Autodesk Inventor part; units mm, degrees
ref_plane "YZ Plane" through (0, 0, 0) normal (1, 0, 0) x (0, 1, 0)
ref_plane "XZ Plane" through (0, 0, 0) normal (0, 1, 0) x (-1, 0, 0)
ref_plane "XY Plane" through (0, 0, 0) normal (0, 0, 1) x (1, 0, 0)
sketch "Szkic1" plane through (0, 0, 0) normal (0, 1, 0) x (-1, 0, 0)
  line L0 (-100, 0) -> (-100, -48)
  line L1 (-11, -7.5) -> (0, -7.5)
  line L2 (-11, -40.5) -> (0, -40.5)
  line L3 (-16, 0) -> (-16, -10.5)
  line L4 (-16, -10.5) -> (-11, -10.5)
  line L5 (-16, -48) -> (-16, -37.5)
  line L6 (-16, -37.5) -> (-11, -37.5)
  line L7 (-11, -21.5) -> (-16, -21.5)
  line L8 (-16, -21.5) -> (-16, -26.5)
  line L9 (-16, -26.5) -> (-11, -26.5)
  line L10 (0, -7.5) -> (0, -14.4549)
  line L11 (0, -40.5) -> (0, -37.5)
  line L12 (0, -7.5) -> (0, -10.5)
  line L13 (0, -10.5) -> (-11, -21.5)
  line L14 (-11, -26.5) -> (0, -37.5)
  line L15 (-100, 0) -> (-100, -48)
  line L16 (-100, 0) -> (-16, 0)
  line L17 (-16, -10.5) -> (-16, 0)
  line L18 (-16, -10.5) -> (-11, -10.5)
  line L19 (-11, -10.5) -> (-11, -7.5)
  line L20 (-11, -7.5) -> (0, -7.5)
  line L21 (0, -7.5) -> (0, -10.5)
  line L22 (0, -10.5) -> (-11, -21.5)
  line L23 (-11, -21.5) -> (-16, -21.5)
  line L24 (-16, -21.5) -> (-16, -26.5)
  line L25 (-16, -26.5) -> (-11, -26.5)
  line L26 (-11, -26.5) -> (0, -37.5)
  line L27 (0, -37.5) -> (0, -40.5)
  line L28 (0, -40.5) -> (-11, -40.5)
  line L29 (-11, -40.5) -> (-11, -37.5)
  line L30 (-11, -37.5) -> (-16, -37.5)
  line L31 (-16, -37.5) -> (-16, -48)
  line L32 (-16, -48) -> (-100, -48)
  line L33 (-100, -48) -> (-100, 0)
  point P0 (0, 0)
  dimension "d1" = 48
  dimension "d2" = 11
  dimension "d5" = 5
  dimension "d6" = 10.5
  dimension "d7" = 10.5
  dimension "d8" = 5
  dimension "d10" = 11
  dimension "d11" = 5
  dimension "d12" = 5
  dimension "d15" = 3
  dimension "d16" = 3
  dimension "d77" = 90
ref_plane "Płaszczyzna konstrukcyjna8" through (100, 0, -48) normal (0, 0, -1) x (-1, 0, 0)
ref_plane "Płaszczyzna konstrukcyjna9" through (100, 0, 0) normal (1, 0, 0) x (0, 0, -1)
sketch "Szkic6" plane through (100, 0, 0) normal (1, 0, 0) x (0, 0, -1)
  line L0 (0, 19) -> (48, 19)
  line L1 (7.5, 19) -> (40.5, 19)
  line L2 (7.5, 19) -> (7.5, 32)
  line L3 (7.5, 32) -> (0, 32)
  line L4 (0, 32) -> (0, 38)
  line L5 (0, 38) -> (10.5, 38)
  line L6 (10.5, 38) -> (10.5, 41)
  line L7 (10.5, 41) -> (7.5, 41)
  line L8 (0, 0) -> (48, 0)
  line L9 (40.5, 19) -> (40.5, 32)
  line L10 (40.5, 32) -> (48, 32)
  line L11 (48, 32) -> (48, 38)
  line L12 (48, 38) -> (37.5, 38)
  line L13 (37.5, 38) -> (37.5, 41)
  line L14 (37.5, 41) -> (40.5, 41)
  line L15 (24.0424, 40.4576) -> (10.5, 54)
  line L16 (23.97, 39) -> (43.1219, 39) construction
  line L17 (24.0424, 40.4576) -> (37.5, 53.9152)
  line L18 (7.5, 41) -> (7.5, 52.5)
  line L19 (7.5, 54) -> (10.5, 54)
  line L20 (37.5, 53.9152) -> (40.5, 53.9152)
  line L21 (40.5, 52.4987) -> (40.5, 41)
  line L22 (23.5, 38) -> (24.5, 38)
  line L23 (23.5, 38) -> (23.5, 41)
  line L24 (24.5, 38) -> (24.5, 41)
  line L25 (7.5, 52.5) -> (7.5, 54)
  line L26 (40.5, 52.4987) -> (40.5, 53.9152)
  point P0 (10.5, 39.5)
  point P1 (24.5, 40.9152)
  point P2 (39, 53.9152)
  dimension "d27" = 33
  dimension "d28" = 7.5
  dimension "d30" = 10.5
  dimension "d32" = 38
  dimension "d33" = 6
  dimension "d36" = 10.5
  dimension "d49" = 3
  dimension "d50" = 3
  dimension "d51" = 135
  dimension "d52" = 1
  dimension "d54" = 3
  dimension "d55" = 13
  dimension "d56" = 3
  dimension "d57" = 3
  dimension "d74" = 53.9152
  dimension "d75" = 13
extrude "Wyciągnięcie proste4" add sketch "Szkic6" against normal blind 50 contours L2 L3 L4 L5 L6 L7 L18 L25 L19 L15 L23 L22 L24 L17 L20 L26 L21 L14 L13 L12 L11 L10 L9 L0
ref_plane "Płaszczyzna konstrukcyjna4" through (0, 0, 0) normal (0, -1, 0) x (1, 0, 0)
sketch "Szkic8" plane through (0, 0, 0) normal (0, -1, 0) x (1, 0, 0)
  line L0 (100, -23.5) -> (50, -23.5)
  point P0 (0, 0)
  point P1 (75, -23.5)
hole "Otwór1" at (75, 0, -23.5) direction (0, 1, 0) diameter 10 end through all
ref_plane "Płaszczyzna konstrukcyjna10" through (100, 19, -40.5) normal (0, 0, -1) x (-1, 0, 0)
sketch "Szkic9" plane through (100, 19, -40.5) normal (0, 0, -1) x (-1, 0, 0)
  line L0 (0, -19) -> (100, -19)
  point P0 (25, 6)
  point P1 (84, -19)
  dimension "d76" = 25
hole "Otwór2" at (75, 25, -40.5) direction (0, 0, 1) diameter 10 end through all
extrude "Wyciągnięcie proste5" add sketch "Szkic1" along normal blind 19
ref_plane "Płaszczyzna konstrukcyjna12" through (0, 19, 0) normal (0, 1, 0) x (1, 0, 0)
sketch "Szkic10" plane through (0, 19, 0) normal (0, 1, 0) x (1, 0, 0)
  line L0 (37, 36.5) -> (37, 11.5) construction
  line L1 (40, 36.5) -> (40, 11.5)
  line L2 (34, 11.5) -> (34, 36.5)
  arc A0 (40, 36.5) -> (34, 36.5) centre (37, 36.5) ccw
  arc A1 (34, 11.5) -> (40, 11.5) centre (37, 11.5) ccw
  line L3 (100, 57.6) -> (100, -9.6)
  line L4 (16, 0) -> (100, 0)
  point P0 (0, 0)
  point P1 (37, 24)
  dimension "d80" = 25
  dimension "d82" = 63
  dimension "d83" = 3
  dimension "d84" = 11.5
extrude "Wyciągnięcie proste6" cut sketch "Szkic10" against normal blind 1
sketch "Szkic11" plane through (16, 0, 0) normal (0, 0, 1) x (1, 0, 0)
  line L0 (34, 19) -> (31, 16)
  line L1 (31, 16) -> (28, 19)
  line L2 (28, 19) -> (34, 19)
  line L3 (84, 19) -> (0, 19)
  point P0 (-16, 0)
  dimension "d89" = 3
extrude "Wyciągnięcie proste7" cut sketch "Szkic11" against normal through all
sketch "Szkic12" plane through (0, 0, 0) normal (0, -1, 0) x (1, 0, 0)
  point P0 (0, 0)
  point P1 (75, -24.5)
hole "Otwór3" at (75, 0, -24.5) direction (0, 1, 0) diameter 10 end through all
Check sheet for the modelled part. Datum: model origin and axes. Units: mm. A direction names the side the tool comes from. Give positions to 0.01 mm unless a question says otherwise; leave off trailing zeros. Write each loop counter-clockwise with the first axis right and the second up, starting at its lowest first coordinate (ties: lowest second). Pieces come first, ordered by that corner, then holes.
Item 1: Scan lines: L1, parallel to Z at x = 14.5, y = 17; L2, parallel to Z at x = 75, y = 5.75; L3, parallel to X at y = 24.5, z = -32. Record each from-to range of solid material in increasing order.
Item 2: Draft check along Z on faces 4 (the face through (75, 47, -40.5)), 5 (the face through (60, 39, -24.5)), 6 (the face through (75, 38, -43)). Enter one of: released by +Z, released by -Z, zero draft, split by the parting line, or undercut.
Item 3: Cross-section at B-B (x = 37). Enter the section's corners in (y, z).
Item 4: Access from +Z, -Z, +X, -X, +Y, -Y to the whole of each face (thin tool, end or side, straight path). Record for faces 1 (the face through (11, 9, -9)), 2 (the face through (16, 9, -24)), 3 (the face through (75, 32, -4)).
Item 5: Cross-section at D-D (y = 22.5). Enter the section's corners in (x, z), and give its area (3 significant figures).
Item 6: Gauge pin test, flat ends, axial feed: pin 1 (1 mm diameter, centred on y = 20, z = -6, fed in from +X); pin 2 (8 mm diameter, centred on x = 62.5, z = -25, fed in from +Y); pin 3 (10 mm diameter, centred on x = 56, y = 45.5, fed in from -Z); pin 4 (1.1 mm diameter, centred on y = 18.5, z = -18.5, fed in from -X). Record the tip position at first contact, or that the pin passes through.
Item 7: Cross-section at C-C (y = 4). Enter the section's corners in (x, z).
Item 8: Cross-section at A-A (y = 17). Enter the section's corners in (x, z).
Report:
1. L1: z = -37.5 to -26.5, -21.5 to -10.5
1. L2: z = -48 to -29.5, -19.5 to 0
1. L3: x = 50 to 70.03, 79.97 to 100
2. face 4: released by -Z
2. face 5: undercut
2. face 6: zero draft
3. outline: (0, -48) - (19, -48) - (19, -39.5) - (18, -39.5) - (18, -8.5) - (19, -8.5) - (19, 0) - (0, 0) - close
4. face 1: +Z, +Y, -Y
4. face 2: -X, +Y, -Y
4. face 3: +Z, +X, -X
5. outline: (50, -40.5) - (70.67, -40.5) - (70.67, -27) arc R5 cw to (70.03, -24) arc R5 cw to (70.67, -21) - (70.67, -7.5) - (50, -7.5) - close; (79.33, -40.5) - (100, -40.5) - (100, -7.5) - (79.33, -7.5) - (79.33, -21) arc R5 cw to (79.97, -24) arc R5 cw to (79.33, -27) - close
5. area: 1,360 mm2
6. pin 1: passes through
6. pin 2: stops at y = 45.42
6. pin 3: stops at z = -40.5
6. pin 4: stops at x = 7.45
7. outline: (0, -40.5) - (11, -40.5) - (11, -37.5) - (16, -37.5) - (16, -48) - (100, -48) - (100, 0) - (16, 0) - (16, -10.5) - (11, -10.5) - (11, -7.5) - (0, -7.5) - (0, -10.5) - (11, -21.5) - (16, -21.5) - (16, -26.5) - (11, -26.5) - (0, -37.5) - close; hole circle Ø10 at (75, -24.5)
8. outline: (0, -40.5) - (11, -40.5) - (11, -37.5) - (16, -37.5) - (16, -48) - (46, -48) - (46, 0) - (16, 0) - (16, -10.5) - (11, -10.5) - (11, -7.5) - (0, -7.5) - (0, -10.5) - (11, -21.5) - (16, -21.5) - (16, -26.5) - (11, -26.5) - (0, -37.5) - close; (48, -48) - (100, -48) - (100, 0) - (48, 0) - close; hole circle Ø10 at (75, -24.5)
